```python
from build123d import *

# Parameters (mm, degrees)
ESQUISSE1_W        = 10.465871206
ESQUISSE1_H        = 10
ESQUISSE1_W_2      = 19.015615649
BOSS_EXTRU_1_DEPTH = 5


with BuildPart() as part:
    # Esquisse1 → Boss.-Extru.1 (new body)
    with BuildSketch(Plane.XY):
        Polygon((90, 82), (90, 167), (90, 172), (80, 172), (80, 167), (10, 167), (10, 172), (0, 172), (0, 167), (0, 0), (0, -5), (5, -5), (5, 0), (60, 0), (60, -5), (70, -5), (70, 0), (90, 0), (90, 44), (75, 44), (75, 82), align=None)
        with Locations((56.967345119, 45)):
            Rectangle(ESQUISSE1_W, ESQUISSE1_H, mode=Mode.SUBTRACT)
        with Locations((56.967345119, 10)):
            Rectangle(ESQUISSE1_W, ESQUISSE1_H, mode=Mode.SUBTRACT)
        with Locations((19.799482129, 35)):
            Rectangle(ESQUISSE1_W_2, ESQUISSE1_H, mode=Mode.SUBTRACT)
    extrude(amount=BOSS_EXTRU_1_DEPTH)


solid = part.part
```
Geometry check sheet. Reference: the model listing, model coordinates, mm. A direction names the side the tool comes from. Give positions to 0.01 mm unless a question says otherwise; leave off trailing zeros. Loops run counter-clockwise (first coordinate to the right, second up) from the corner with the lowest first, then second, coordinate; pieces in that order, holes last. Notation, with made-up numbers: M 72.25,14 L 115.25,14 A12 ccw 115.25,20 Z; hole C 24.5,4 d7. An arc over 180 degrees is marked long. Write item = value, one per line. Start each with the question number.
1. Thickness scan on probe 1 along Y at (x, z) = (21.5, 2.3); probe 2 along Y at (x, z) = (55.5, 0.6); probe 3 along Y at (x, z) = (51, 1.8). Record the ranges inside material, lowest first.
2. Section check B-B, the plane z = 0.75. Give the number of separate pieces and of enclosed holes in the cut face, plus the area to 3 significant figures.
3. Section check A-A, the plane x = 26.5. Enter the section's corners in (y, z).
4. Draft check along X on faces 4 (the face through (10.292, 35, 2)), 5 (the face through (90, 22, 2)), 6 (the face through (82, 82, 2)), 7 (the face through (0, 85, 2)). Enter one of: +X half, -X half, draft (parallel to the pull), parting line (faces both ways), or undercut.
5. Go/stop test with flat-tipped pins: P1, Ø2.5, axis at y = 45, z = 2.5, coming from the -X side; P2, Ø1.5, axis at y = -2.5, z = 3.5, coming from the +X side; P3, Ø2.5, axis at x = 75, z = 1.5, coming from the -Y side; P4, Ø2.5, axis at y = 62.5, z = 3.5, coming from the +X side. Record where each tip stops, or that it passes through.
6. Section check D-D, the plane y = 63.5. Enter the section's corners in (x, z), plus the area to 3 significant figures.
7. Section check C-C, the plane y = 10. Enter the section's corners in (x, z), plus the area to 3 significant figures.
8. Tool access check on faces 1 (the face through (20, 30, 2)), 2 (the face through (80, 170, 2)), 3 (the face through (80, 0, 2)). Record the directions out of +Z, -Z, +X, -X, +Y, -Y that give a thin tool (end or side, any length) a straight path to the whole face; none if there is none.
Values follow:
q1.probe_1 = 0 to 30, 40 to 167
q1.probe_2 = 0 to 5, 15 to 40, 50 to 167
q1.probe_3 = 0 to 167
q2.separate_pieces = 1
q2.enclosed_holes = 3
q2.area = 14,200 mm^2
q3.outline = M 0,0 L 30,0 L 30,5 L 0,5 Z; M 40,0 L 167,0 L 167,5 L 40,5 Z
q4.face_4 = undercut
q4.face_5 = +X half
q4.face_6 = draft
q4.face_7 = -X half
q5.P1 = 0
q5.P2 = 70
q5.P3 = 0
q5.P4 = 75
q6.outline = M 0,0 L 75,0 L 75,5 L 0,5 Z
q6.area = 375 mm^2
q7.outline = M 0,0 L 51.73,0 L 51.73,5 L 0,5 Z; M 62.2,0 L 90,0 L 90,5 L 62.2,5 Z
q7.area = 398 mm^2
q8.face_1 = +Z, -Z
q8.face_2 = +Z, -Z, +Y
q8.face_3 = +Z, -Z, +X, -Y
